Geometry: see drawing. Coordinates: mm, zero at the bounding-box minimum. A direction names the side the tool comes from. Round coordinates to 2 decimals unless told otherwise and drop trailing zeros. Order: outer loops, then holes, each group sorted by start corner. A loop starts at its lowest first (then second) coordinate and runs counter-clockwise, first axis right, second up. Notation, with made-up numbers: (50.25, 82.5) -> (103.25, 82.5) arc R16 cw to (103.25, 104.5) -> close; hole circle Ø6 at (-27, -17). An arc over 180 degrees is marked (long way). One line per item, written item: value. Start each with the question number.
1) Section B-B (y = 66). Return the cut outline in (x, z), and give its area (3 significant figures).
2) Section D-D (x = 7.5). Return the cut outline in (y, z).
3) Mould query, pull axis X, two halves, no side actions, for the marked faces 1, 2 and 3. Classes: pulls with the +X half, pulls with the -X half, needs draft (parallel to the pull), parting line crosses it, or undercut.
4) Reachability of the marked faces 4 and 5 from +Z, -Z, +X, -X, +Y, -Y: full face, straight path, thin tool, end or side. Return the list, or none.
5) Ray query, L1, parallel to Y at x = 18, z = 18; L2, parallel to Z at x = 40, y = 35.5; L3, parallel to X at y = 8, z = 40. Return the intervals inside material, ascending.
6) Section A-A (x = 40). Return the cut outline in (y, z).
7) Pin query (flat end, axial travel): P1, Ø12, axis at x = 24, y = 46.5, coming from the +Z side; P2, Ø2, axis at x = 64, y = 11, coming from the +Z side (1 decimal); P3, Ø10, axis at x = 37.5, y = 16.5, coming from the +Z side. Return the tip coordinate at first contact, or that it passes through.
8) Section C-C (z = 40). Return the cut outline in (x, y), and give its area (3 significant figures).
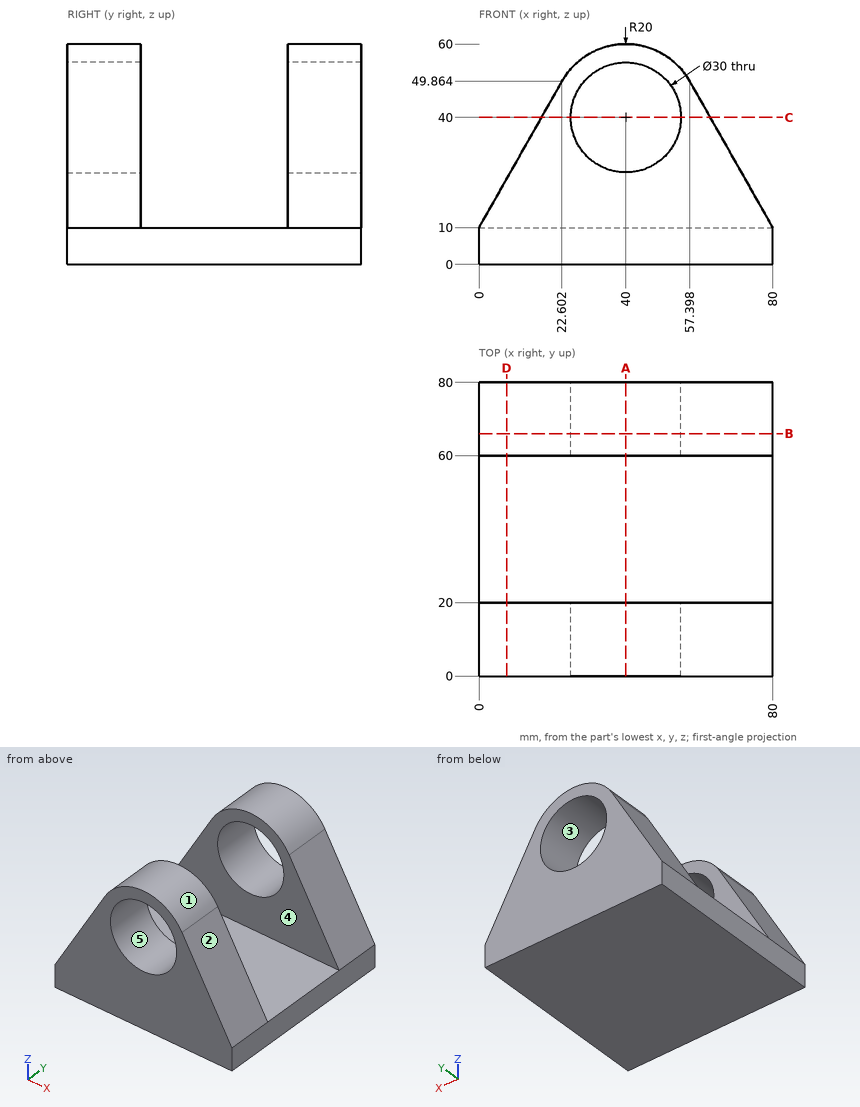
Findings:
1. outline: (0, 0) -> (80, 0) -> (80, 10) -> (57.4, 49.86) arc R20 ccw to (22.6, 49.86) -> (0, 10) -> close; hole circle Ø30 at (40, 40)
1. area: 2,630 mm2
2. outline: (0, 0) -> (80, 0) -> (80, 23.23) -> (60, 23.23) -> (60, 10) -> (20, 10) -> (20, 23.23) -> (0, 23.23) -> close
3. face 1: parting line crosses it
3. face 2: pulls with the +X half
3. face 3: undercut
4. face 4: +Z, +X, -X
4. face 5: +Y, -Y
5. L1: 0 to 20, 60 to 80
5. L2: 0 to 10
5. L3: 17.01 to 25, 55 to 62.99
6. outline: (0, 0) -> (80, 0) -> (80, 25) -> (60, 25) -> (60, 10) -> (20, 10) -> (20, 25) -> (0, 25) -> close; (0, 55) -> (20, 55) -> (20, 60) -> (0, 60) -> close; (60, 55) -> (80, 55) -> (80, 60) -> (60, 60) -> close
7. P1: z = 10
7. P2: z = 40
7. P3: z = 60
8. outline: (17.01, 0) -> (25, 0) -> (25, 20) -> (17.01, 20) -> close; (17.01, 60) -> (25, 60) -> (25, 80) -> (17.01, 80) -> close; (55, 0) -> (62.99, 0) -> (62.99, 20) -> (55, 20) -> close; (55, 60) -> (62.99, 60) -> (62.99, 80) -> (55, 80) -> close
8. area: 639 mm2
